```python
from build123d import *

# Parameters (mm, degrees)
F0_W           = 371.3734
F0_H           = 18.415
F1_DEPTH       = 44.45
F5_D           = 6.35
F5_DEPTH       = 12.7
F5_TIP         = 1.9077324654
F5_ON_F3_D     = 6.35
F5_ON_F3_DEPTH = 12.7
F5_ON_F3_TIP   = 1.9077324654
F5_ON_F2_D     = 6.35
F5_ON_F2_DEPTH = 12.7
F5_ON_F2_TIP   = 1.9077324654


with BuildPart() as f1:
    # F0 (on Front) → F1 (new body)
    with BuildSketch(Plane.XZ):
        with Locations((73.7288090025, -9.8947464747)):
            Rectangle(F0_W, F0_H)
    extrude(amount=F1_DEPTH)

    # F5
    with Locations(Plane(origin=(-111.9578909975, 0, 0), x_dir=(0, -1, 0), z_dir=(-1, 0, 0))):
        with Locations((7.62, -10.2122464747), (36.83, -10.2122464747)):
            Hole(F5_D / 2, depth=F5_DEPTH)
            with Locations((0, 0, -(F5_DEPTH + F5_TIP / 2))):  # 118° drill point
                Cone(0, F5_D / 2, F5_TIP, mode=Mode.SUBTRACT)

    # F5 on F3
    with Locations(Plane.YZ.offset(259.4155090025)):
        with Locations((-36.83, -10.2122464747)):
            Hole(F5_ON_F3_D / 2, depth=F5_ON_F3_DEPTH)
            with Locations((0, 0, -(F5_ON_F3_DEPTH + F5_ON_F3_TIP / 2))):  # 118° drill point
                Cone(0, F5_ON_F3_D / 2, F5_ON_F3_TIP, mode=Mode.SUBTRACT)

    # F5 on F2
    with Locations(Plane.YZ.offset(259.4155090025)):
        with Locations((-7.62, -10.2122464747)):
            Hole(F5_ON_F2_D / 2, depth=F5_ON_F2_DEPTH)
            with Locations((0, 0, -(F5_ON_F2_DEPTH + F5_ON_F2_TIP / 2))):  # 118° drill point
                Cone(0, F5_ON_F2_D / 2, F5_ON_F2_TIP, mode=Mode.SUBTRACT)


solid = f1.part
```
Input: part model. Units: mm. Frame: model coordinates. A direction names the side the tool comes from. Coordinates: 2 decimals unless noted, no trailing zeros.
Q1. Set-up query: faces 1 (the cylindrical face through (252.977, -9.327, -7.535)), 2 (the cylindrical face through (-105.5, -39.2, -8.1)), 3 (the flat face through (71, 0, -10)). Return all of +Z, -Z, +X, -X, +Y, -Y with unobstructed straight access to the full face (end or side cutting, diameter ignored); none if empty.
Results are:
face 1: +X
face 2: -X
face 3: +Z, -Z, +X, -X, +Y
Q2. Contact query for flat-ended pins moving along their axis: pin 1 (4 mm diameter, centred on y = -36.83, z = -10.21, fed in from +X); pin 2 (5 mm diameter, centred on y = -36.83, z = -10.21, fed in from +X). Output: stop coordinate, or through.
Results are:
pin 1: stops at x = 246.01
pin 2: stops at x = 246.31
Q3. Mould query, pull axis Z, two halves, no side actions, for faces 4 (the flat face through (71, -22, -19.102)), 5 (the flat face through (-111.958, -22, -10)), 6 (the cylindrical face through (-105.519, -9.96, -8.066)). Classes: +Z half, -Z half, draft (parallel to the pull), parting line (faces both ways), or undercut.
Results are:
face 4: -Z half
face 5: draft
face 6: undercut
Q4. Line query: line 1 along Z through (x, y) = (-105.25, -7.62); line 2 along Z through (x, y) = (253, -7); line 3 along X through (y, z) = (-37, -13). Output: solid intervals per line, ascending.
Results are:
line 1: z = -19.1 to -13.39, -7.04 to -0.69
line 2: z = -19.1 to -13.33, -7.1 to -0.69
line 3: x = -99.03 to 246.49
